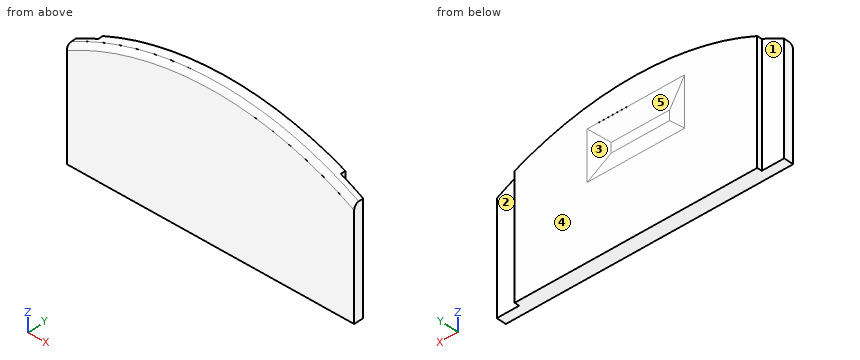
```python
from build123d import *

# Parameters (mm, degrees)
BOSS_EXTRUDE1_DEPTH = 19.05
SKETCH2_W           = 12.7
SKETCH2_H           = 6.35
CUT_EXTRUDE1_DEPTH  = 0.635
CHAMFER1_SIZE       = 2.54
CHAMFER1_SIZE2      = 0.633293127
CUT_EXTRUDE2_DEPTH  = 27.785034651
FILLET1_R           = 0.635


with BuildPart() as part:
    # Sketch1 → Boss-Extrude1 (new body)
    with BuildSketch(Plane.XY):
        Polygon((-18.7325, 0), (18.7325, 0), (18.7325, 1.27), (15.8115, 1.27), (15.8115, 1.905), (-15.8115, 1.905), (-15.8115, 1.27), (-18.7325, 1.27), align=None)
    extrude(amount=BOSS_EXTRUDE1_DEPTH)

    # Sketch2 → Cut-Extrude1 (cut)
    with BuildSketch(Plane(origin=(0, 1.905, 0), x_dir=(1, 0, 0), z_dir=(0, 1, 0))):
        with Locations((0, -12.7)):
            Rectangle(SKETCH2_W, SKETCH2_H)
    extrude(amount=-CUT_EXTRUDE1_DEPTH, mode=Mode.SUBTRACT)

    # Chamfer1
    chamfer1_edges = [part.edges().sort_by_distance(p)[0] for p in [
        (6.35, 1.27, 12.7),
        (0, 1.27, 15.875),
        (-6.35, 1.27, 12.7),
        (0, 1.27, 9.525),
    ]]
    chamfer1_side = [part.faces().sort_by_distance(p)[0] for p in [
        (0, 1.27, 12.7),
    ]]
    chamfer(chamfer1_edges, length=CHAMFER1_SIZE, length2=CHAMFER1_SIZE2, reference=chamfer1_side[0])

    # Sketch3 → Cut-Extrude2 (cut, through all)
    with BuildSketch(Plane(origin=(0, 1.905, 0), x_dir=(1, 0, 0), z_dir=(0, 1, 0))):
        with BuildLine():
            Line((-18.7325, -21.59), (18.7325, -21.59))
            Line((18.7325, -21.59), (18.7325, -14.233613746))
            ThreePointArc((18.7325, -14.233613746), (0, -19.05), (-18.7325, -14.233613746))
            Line((-18.7325, -14.233613746), (-18.7325, -21.59))
        make_face()
    extrude(amount=-CUT_EXTRUDE2_DEPTH, mode=Mode.SUBTRACT)

    # Fillet1
    fillet1_edges = [part.edges().sort_by_distance(p)[0] for p in [
        (0, 0, 19.05),
    ]]
    fillet(fillet1_edges, radius=FILLET1_R)


solid = part.part
```
The listing builds one solid part. Answer for the finished solid, in the listing's coordinates (mm). Face numbers are marked on the shaded views. A direction names the side the tool comes from. Give positions to 0.01 mm unless a question says otherwise; leave off trailing zeros. Order: outer loops, then holes, each group sorted by start corner. A loop starts at its lowest first (then second) coordinate and runs counter-clockwise, first axis right, second up. Notation, with made-up numbers: (-36.75, 10.5) - (10.25, 10.5) arc R11 cw to (10.25, 26.5) - close; hole circle Ø9 at (8, 55). An arc over 180 degrees is marked (long way). Answer in a Markdown table with one row per item. Add a question column.
Q1. The part is cut by section C-C (y = 0.3). Determine the outline of the cut face in (x, z), then the cut area to 3 significant figures.
Q2. The part is cut by section A-A (z = 6.75). Determine the outline of the cut face in (x, y) (1 decimal).
Q3. Given P1, Ø5, axis at x = -7.5, z = 9, coming from the -Y side; P2, Ø0.9, axis at x = -17, z = 10.5, coming from the +Y side, each flat-ended and moving along its own axis, determine where each tip first touches the part or whether it passes through.
Q4. Which of the six approach directions +Z, -Z, +X, -X, +Y, -Y give full straight-line access (tool end or side, diameter ignored) to the marked faces 1, 2 and 3?
Q5. Find the intervals of material crossed by line 1 along X through (y, z) = (1.35, 8.25); line 2 along Z through (x, y) = (-5, 1.1); line 3 along Z through (x, y) = (1, 1.1), in increasing order. Write a range as [from, to].
Q6. For a pull along X with two mould halves and no side action, classify the marked faces 4 and 5 as released by +X, released by -X, zero draft, split by the parting line, or undercut.
Determined:
| question | item | result |
|---|---|---|
| 1 | outline | (-18.73, 0) - (18.73, 0) - (18.73, 14.12) arc R38.74 ccw to (-18.73, 14.12) - close |
| 1 | area | 651 mm² |
| 2 | outline | (-18.7, 0) - (18.7, 0) - (18.7, 1.3) - (15.8, 1.3) - (15.8, 1.9) - (-15.8, 1.9) - (-15.8, 1.3) - (-18.7, 1.3) - close |
| 3 | P1 | stops at y = 0 |
| 3 | P2 | stops at y = 1.27 |
| 4 | face 1 | +Z, -Z, -X, +Y |
| 4 | face 2 | +Z, -Z, +X, +Y |
| 4 | face 3 | +Y |
| 5 | line 1 | x = [-15.81, 15.81] |
| 5 | line 2 | z = [0, 18.73] |
| 5 | line 3 | z = [0, 19.04] |
| 6 | face 4 | zero draft |
| 6 | face 5 | undercut |
